from build123d import *

# Parameters (mm, degrees)
F1_DEPTH      = 150
F1_DEPTH_BACK = 150
F0_W          = 49.675524
F0_H          = 124.247186
F2_DEPTH      = 120
F2_DEPTH_BACK = 120
F4_D          = 50
F5_D          = 50


with BuildPart() as f1:
    # F0 (on Front) → F1 (new body, two sides)
    with BuildSketch(Plane.XZ) as f1_sk:
        with BuildLine():
            Line((-39.200012, 62.123593), (-70.046909, 62.123593))
            ThreePointArc((-70.046909, 62.123593), (0, 0.094575), (70.046909, 62.123593))
            Line((70.046909, 62.123593), (39.200012, 62.123593))
            Line((39.200012, 62.123593), (39.200012, 26.869994))
            Line((39.200012, 26.869994), (-39.200012, 26.869994))
            Line((-39.200012, 26.869994), (-39.200012, 62.123593))
        make_face()
        with BuildLine():
            ThreePointArc((39.200012, 62.123593), (0, 27.270557), (-39.200012, 62.123593))
            Line((-39.200012, 62.123593), (-39.200012, 26.869994))
            Line((-39.200012, 26.869994), (39.200012, 26.869994))
            Line((39.200012, 26.869994), (39.200012, 62.123593))
        make_face()
    extrude(amount=F1_DEPTH)
    extrude(f1_sk.sketch, amount=-F1_DEPTH_BACK)

    # F0 (on Front) → F2 (join, two sides)
    with BuildSketch(Plane.XZ) as f2_sk:
        with Locations((-94.884671, 0)):
            Rectangle(F0_W, F0_H)
        with BuildLine():
            ThreePointArc((70.046909, 62.123593), (0, 0.094575), (-70.046909, 62.123593))
            Line((-70.046909, 62.123593), (-70.046909, -62.123593))
            Line((-70.046909, -62.123593), (70.046909, -62.123593))
            Line((70.046909, -62.123593), (70.046909, 62.123593))
        make_face()
        with Locations((94.884671, 0)):
            Rectangle(F0_W, F0_H)
    extrude(amount=F2_DEPTH)
    extrude(f2_sk.sketch, amount=-F2_DEPTH_BACK)

    # F4 (through all)
    with Locations(Plane.XY):
        with Locations((-84.698744, 0), (81.866011, 0)):
            Hole(F4_D / 2)

    # F5 (through all)
    with Locations(Plane(origin=(0, 0, 0), x_dir=(1, 0, 0), z_dir=(0, 0, -1))):
        with Locations((-84.698744, 0), (81.866011, 0)):
            Hole(F5_D / 2)


solid = f1.part
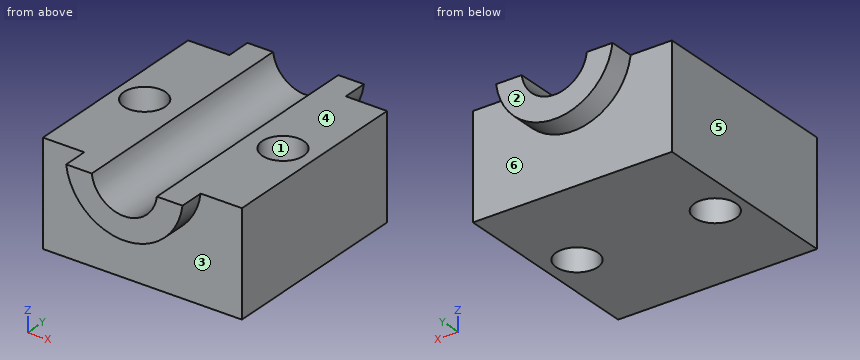
Design review of the part built by this model. Coordinates are the model's own, in mm. Face numbers are marked on the shaded views. A direction names the side the tool comes from. Give positions to 0.01 mm unless a question says otherwise; leave off trailing zeros. Order: outer loops, then holes, each group sorted by start corner. A loop starts at its lowest first (then second) coordinate and runs counter-clockwise, first axis right, second up.
1. To check wall thickness, follow L1, parallel to Y at x = -83, z = -0.5; L2, parallel to Y at x = 68, z = -32.5; L3, parallel to Y at x = -13, z = -12.5. State the ranges of each line that lie inside material, in increasing order.
Solution:
L1: y = -120 to -24.94, 24.94 to 120
L2: y = -120 to -20.8, 20.8 to 120
L3: y = -120 to 120
2. Mouldability with a two-part tool opening along Y and no side actions: class the marked faces 1, 2, 3 and 4 as +Y half, -Y half, draft (parallel to the pull), parting line (faces both ways), or undercut.
Solution:
face 1: undercut
face 2: +Y half
face 3: -Y half
face 4: draft
3. Add section C-C, the plane x = -85. State the section outline as (y, z) points.
Solution:
outline: (-120, -62.12) - (-25, -62.12) - (-25, 62.12) - (-120, 62.12) - close; (25, -62.12) - (120, -62.12) - (120, 62.12) - (25, 62.12) - close
4. Add section A-A, the plane y = 0. State the section outline as (x, z) points.
Solution:
outline: (-119.72, -62.12) - (-109.7, -62.12) - (-109.7, 62.12) - (-119.72, 62.12) - close; (-59.7, -62.12) - (56.87, -62.12) - (56.87, 62.12) - (39.2, 62.12) arc R39.47 cw to (-39.2, 62.12) - (-59.7, 62.12) - close; (106.87, -62.12) - (119.72, -62.12) - (119.72, 62.12) - (106.87, 62.12) - close
5. Add section D-D, the plane z = -45. State the section outline as (x, y) points.
Solution:
outline: (-119.72, -120) - (119.72, -120) - (119.72, 120) - (-119.72, 120) - close; hole circle Ø50 at (-84.7, 0); hole circle Ø50 at (81.87, 0)
6. Add section B-B, the plane z = 49. State the section outline as (x, y) points.
Solution:
outline: (-119.72, -120) - (-67.16, -120) - (-67.16, -150) - (-35.26, -150) - (-35.26, 150) - (-67.16, 150) - (-67.16, 120) - (-119.72, 120) - close; (35.26, -150) - (67.16, -150) - (67.16, -120) - (119.72, -120) - (119.72, 120) - (67.16, 120) - (67.16, 150) - (35.26, 150) - close; hole circle Ø50 at (-84.7, 0); hole circle Ø50 at (81.87, 0)
7. For pin 1 Ø12 at (x, z) = (-22, -48.5) entering from +Y, flat-tipped, find the tip position at first contact; note if it passes through.
Solution:
pin 1: stops at y = 120
8. Tool access review of the marked faces 5 and 6: name each direction out of +Z, -Z, +X, -X, +Y, -Y from which nothing blocks a thin tool from reaching the whole face with its end or side.
Solution:
face 5: +Z, -Z, -X, +Y, -Y
face 6: -Z, +Y
